For this review, use the dimensioned drawing (mm, ordinates from the lowest corner) and the shaded views. A direction names the side the tool comes from. Coordinates: 2 decimals unless noted, no trailing zeros. Loops run counter-clockwise (first coordinate to the right, second up) from the corner with the lowest first, then second, coordinate; pieces in that order, holes last.
1. To check wall thickness, follow probe 1 along Y at (x, z) = (5, 1.8); probe 2 along Z at (x, y) = (1.75, 5.5); probe 3 along X at (y, z) = (6.25, 1.25). State the ranges of each line that lie inside material, in increasing order.
2. Take a section at A-A, the plane z = 4. State the section outline as (x, y) points.
3. Take a section at D-D, the plane x = 3.75. State the section outline as (y, z) points (3 decimals).
4. Clearance check with flat-ended pins moving along their axes: P1, Ø1.2, axis at y = 5, z = 1.5, coming from the -X side; P2, Ø0.6, axis at x = 2, y = 5, coming from the -Z side; P3, Ø1.2, axis at x = 3.5, y = 5.5, coming from the +Z side (3 decimals). State where each tip first meets the part, or that it passes through.
5. Machinability: for the marked faces 1, 2, 3 and 4, which of the approach directions +Z, -Z, +X, -X, +Y, -Y give a long, thin tool a straight path to every point of the face, cutting with its end or side? Answer none if there is none.
6. Take a section at C-C, the plane y = 5.5. State the section outline as (x, z) points (3 decimals), then the cut area to 3 significant figures.
7. Take a section at B-B, the plane x = 6.5. State the section outline as (y, z) points.
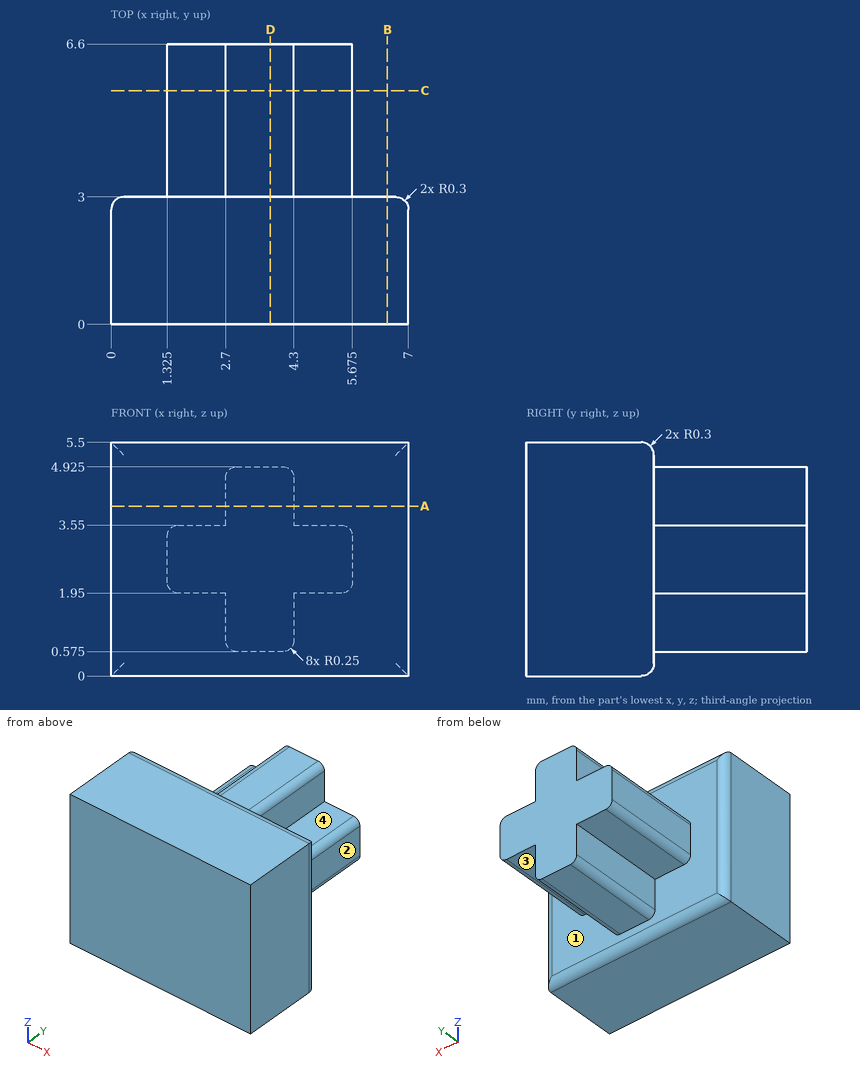
Results list:
1. probe 1: y = 0 to 3
1. probe 2: z = 1.95 to 3.55
1. probe 3: x = 2.7 to 4.3
2. outline: (0, 0) - (7, 0) - (7, 2.7) arc R0.3 ccw to (6.7, 3) - (4.3, 3) - (4.3, 6.6) - (2.7, 6.6) - (2.7, 3) - (0.3, 3) arc R0.3 ccw to (0, 2.7) - close
3. outline: (0, 0) - (2.7, 0) arc R0.3 ccw to (3, 0.3) - (3, 0.575) - (6.6, 0.575) - (6.6, 4.925) - (3, 4.925) - (3, 5.2) arc R0.3 ccw to (2.7, 5.5) - (0, 5.5) - close
4. P1: stops at x = 1.35
4. P2: stops at z = 1.95
4. P3: stops at z = 4.925
5. face 1: +Y
5. face 2: +Z, -Z, +X, +Y
5. face 3: -Z, +X, +Y
5. face 4: +Z, +X, +Y
6. outline: (1.325, 2.2) arc R0.25 ccw to (1.575, 1.95) - (2.7, 1.95) - (2.7, 0.825) arc R0.25 ccw to (2.95, 0.575) - (4.05, 0.575) arc R0.25 ccw to (4.3, 0.825) - (4.3, 1.95) - (5.425, 1.95) arc R0.25 ccw to (5.675, 2.2) - (5.675, 3.3) arc R0.25 ccw to (5.425, 3.55) - (4.3, 3.55) - (4.3, 4.675) arc R0.25 ccw to (4.05, 4.925) - (2.95, 4.925) arc R0.25 ccw to (2.7, 4.675) - (2.7, 3.55) - (1.575, 3.55) arc R0.25 ccw to (1.325, 3.3) - close
6. area: 11.3 mm2
7. outline: (0, 0) - (2.7, 0) arc R0.3 ccw to (3, 0.3) - (3, 5.2) arc R0.3 ccw to (2.7, 5.5) - (0, 5.5) - close
